from build123d import *

# Parameters (mm, degrees)
F0_R     = 7.6
F0_R_2   = 4
F1_DEPTH = 50
F2_DEPTH = 25


with BuildPart() as f1:
    # F0 (on Top) → F1 (new body)
    with BuildSketch(Plane.XY):
        with Locations((-47.129215, 0)):
            Circle(F0_R)
        with Locations((-47.129215, 0)):
            Circle(F0_R_2, mode=Mode.SUBTRACT)
        with Locations((-47.129215, 0)):
            Circle(F0_R_2)
    extrude(amount=-F1_DEPTH)

    # F0 (on Top) → F2 (join)
    with BuildSketch(Plane.XY):
        with Locations((-47.129215, 0)):
            Circle(F0_R_2)
    extrude(amount=F2_DEPTH)


with BuildPart() as f1_1:
    # F3: moved
    add(f1.part.moved(Location((0, -5, 25))))


solid = f1_1.part
Design review of the part built by this model. Coordinates are the model's own, in mm. A direction names the side the tool comes from. Coordinates: 2 decimals unless noted, no trailing zeros. Loops run counter-clockwise (first coordinate to the right, second up) from the corner with the lowest first, then second, coordinate; pieces in that order, holes last. Notation, with made-up numbers: (37, -13) -> (89, -13) arc R27 ccw to (89, 23) -> close; hole circle Ø10 at (26.5, -26). An arc over 180 degrees is marked (long way). Use a Markdown table: item, result. Add a question column.
Item 1: We need section B-B, the plane x = -47. Write out the cut boundary in (y, z).
Item 2: Clearance check with flat-ended pins moving along their axes: P1, Ø8, axis at x = -49, z = 30.5, coming from the +Y side; P2, Ø1, axis at x = -49.5, y = -11, coming from the +Z side; P3, Ø3, axis at y = 0, z = 34, coming from the +X side. State where each tip first meets the part, or that it passes through.
Item 3: Machinability: for faces 1 (the flat face through (-44, -8, 25)), 2 (the cylindrical face through (-54.722, -4.666, 0.35)), which of the approach directions +Z, -Z, +X, -X, +Y, -Y give a long, thin tool a straight path to every point of the face, cutting with its end or side? Answer none if there is none.
Item 4: We need section D-D, the plane z = 32. Write out the cut boundary in (x, y).
Item 5: Wall thickness on L1, parallel to Z at x = -45.5, y = 0.5; L2, parallel to Y at x = -44, z = 16; L3, parallel to Y at x = -44.25, z = 12: over which ranges is each line inside the solid? List them lowest first. Write a range as from..to.
Item 6: We need section A-A, the plane y = -5. Write out the cut boundary in (x, z).
Item 7: We need section C-C, the plane z = -13. Write out the cut boundary in (x, y), and give its area (3 significant figures).
Numbers:
| question | item | result |
|---|---|---|
| 1 | outline | (-12.6, -25) -> (2.6, -25) -> (2.6, 25) -> (-1, 25) -> (-1, 50) -> (-9, 50) -> (-9, 25) -> (-12.6, 25) -> close |
| 2 | P1 | stops at y = -1 |
| 2 | P2 | stops at z = 25 |
| 2 | P3 | stops at x = -45.19 |
| 3 | face 1 | +Z |
| 3 | face 2 | +Z, -Z |
| 4 | outline | circle Ø8 at (-47.13, -5) |
| 5 | L1 | z = -25..25 |
| 5 | L2 | y = -11.93..1.93 |
| 5 | L3 | y = -12.03..2.03 |
| 6 | outline | (-54.73, -25) -> (-39.53, -25) -> (-39.53, 25) -> (-43.13, 25) -> (-43.13, 50) -> (-51.13, 50) -> (-51.13, 25) -> (-54.73, 25) -> close |
| 7 | outline | circle Ø15.2 at (-47.13, -5) |
| 7 | area | 181 mm^2 |
